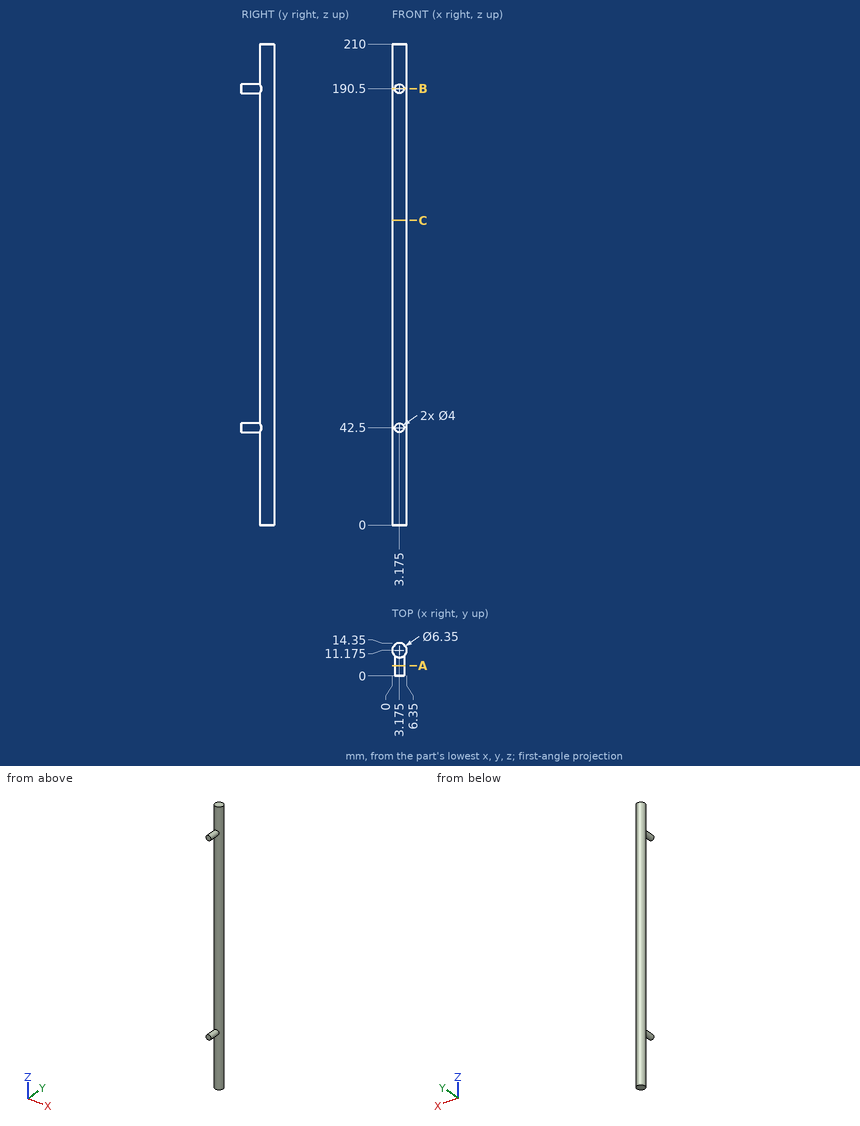
Input: dimensioned drawing with shaded views. Units: mm. Origin: part minimum x, y, z. Coordinates: 2 decimals unless noted, no trailing zeros. Order: outer loops, then holes, each group sorted by start corner. A loop starts at its lowest first (then second) coordinate and runs counter-clockwise, first axis right, second up.
1. Ray query, line 1 along Z through (x, y) = (4, 2.75); line 2 along Y through (x, z) = (3.5, 169.5); line 3 along X through (y, z) = (11.5, 117.5). Return the intervals inside material, ascending.
Checked values:
line 1: z = 40.68 to 44.32, 188.68 to 192.32
line 2: y = 8.02 to 14.33
line 3: x = 0.02 to 6.33
2. Cut plane B-B, the plane z = 190.5. Return loops of the section in (x, y) (3 decimals).
Checked values:
outline: (1.175, 0) - (5.175, 0) - (5.175, 8.709) arc R3.175 ccw (long way) to (1.175, 8.709) - close
3. Cut plane A-A, the plane y = 4.5. Return loops of the section in (x, z) (3 decimals), plus the area to 3 significant figures.
Checked values:
outline: circle Ø4 at (3.175, 42.5); circle Ø4 at (3.175, 190.5)
area: 25.1 mm2
4. Contact query for flat-ended pins moving along their axis: P1, Ø2, axis at x = 3, z = 122.5, coming from the +Y side; P2, Ø1.5, axis at x = 5.5, z = 33, coming from the +Y side; P3, Ø1, axis at x = 5.5, z = 156.5, coming from the +Y side. Output: stop coordinate, or through.
Checked values:
P1: stops at y = 14.35
P2: stops at y = 13.93
P3: stops at y = 13.77
5. Cut plane C-C, the plane z = 133. Return loops of the section in (x, y) (3 decimals), plus the area to 3 significant figures.
Checked values:
outline: circle Ø6.35 at (3.175, 11.175)
area: 31.7 mm2
